```python
from build123d import *

# Parameters (mm, degrees)
SM_BASE_FLANGE_1_DEPTH = 113
EXTRUDE_1_DEPTH        = 4
HOLE_WIZARD_M3_1_D     = 2.5
SKETCH_11_W            = 71.5874944
SKETCH_11_H            = 95.16
CUT_EXTRUDE_1_DEPTH    = 44
HOLE_WIZARD_M3_2_D     = 2.5


# Sheet-metal steps are written as plain solids
with BuildPart() as part:
    # Sketch 2 → 基体-法兰1 (new body)
    with BuildSketch(Plane.XY):
        with BuildLine():
            Line((74, 45.58), (1.5, 45.58))
            ThreePointArc((1.5, 45.58), (0.439339828, 45.140660172), (0, 44.08))
            Line((0, 44.08), (0, -44.08))
            ThreePointArc((0, -44.08), (0.439339828, -45.140660172), (1.5, -45.58))
            Line((1.5, -45.58), (74, -45.58))
            Line((74, -45.58), (74, -47.58))
            Line((74, -47.58), (1.5, -47.58))
            ThreePointArc((1.5, -47.58), (-0.974873734, -46.554873734), (-2, -44.08))
            Line((-2, -44.08), (-2, 44.08))
            ThreePointArc((-2, 44.08), (-0.974873734, 46.554873734), (1.5, 47.58))
            Line((1.5, 47.58), (74, 47.58))
            Line((74, 47.58), (74, 45.58))
        make_face()
    extrude(amount=-SM_BASE_FLANGE_1_DEPTH)

    # 草图7 → 凸台-拉伸1 (add)
    with BuildSketch(Plane.XY):
        with BuildLine():
            Line((74, 45.58), (1.5, 45.58))
            ThreePointArc((1.5, 45.58), (0.439339828, 45.140660172), (0, 44.08))
            Line((0, 44.08), (0, -44.08))
            ThreePointArc((0, -44.08), (0.439339828, -45.140660172), (1.5, -45.58))
            Line((1.5, -45.58), (74, -45.58))
            Line((74, -45.58), (74, 45.58))
        make_face()
    extrude(amount=-EXTRUDE_1_DEPTH)

    # M3 螺纹孔1 (through all)
    with Locations(Plane(origin=(0, 47.58, 0), x_dir=(1, 0, 0), z_dir=(0, 1, 0))):
        with Locations((53.7, 100.6), (66.2, 100.6)):
            Hole(HOLE_WIZARD_M3_1_D / 2)

    # 草图11 → 切除-拉伸1 (cut)
    with BuildSketch(Plane.ZY.offset(2)):
        with Locations((-91.7937472, 0)):
            Rectangle(SKETCH_11_W, SKETCH_11_H)
    extrude(amount=-CUT_EXTRUDE_1_DEPTH, mode=Mode.SUBTRACT)

    # M3 螺纹孔2 (through all)
    with Locations(Plane(origin=(0, 0, -4), x_dir=(-1, 0, 0), z_dir=(0, 0, -1))):
        with Locations((-51.5, 12.5), (-26.5, 12.5), (-26.5, -12.5), (-51.5, -12.5)):
            Hole(HOLE_WIZARD_M3_2_D / 2)


solid = part.part
```
Can you work these out from the model? Positions are in its coordinate system, mm. A direction names the side the tool comes from. Round coordinates to 2 decimals unless told otherwise and drop trailing zeros. Loops run counter-clockwise (first coordinate to the right, second up) from the corner with the lowest first, then second, coordinate; pieces in that order, holes last.
Item 1: If we mould it in two halves opening along X, with no side actions, what happens to faces 4 (the flat face through (74, 0, -2)), 5 (the cylindrical face through (65.623, 46.566, -99.491)), 6 (the cylindrical face through (-1, 46.53, -27.61))? For each: +X half, -X half, draft (parallel to the pull), parting line (faces both ways), or undercut.
Item 2: Suppose I cut it at C-C, the plane y = -39. Write out the boundary of the cut face in (x, z), then the cut area to 3 significant figures.
Item 3: Suppose I cut it at D-D, the plane x = 3. Write out the boundary of the cut face in (y, z).
Item 4: Which directions (+Z, -Z, +X, -X, +Y, -Y) give clear straight access to the entire face, cutting with the end or side of a thin tool? Please do faces 1 (the flat face through (36, 1, -4)), 2 (the flat face through (35, 1, 0)), 3 (the flat face through (-1, 0, -56)).
Item 5: Suppose I cut it at A-A, the plane z = -51. Write out the boundary of the cut face in (x, y), then the cut area to 3 significant figures.
Item 6: Please list where these lines run through material, in increasing order: L1, parallel to Y at x = 51.5, z = -2.7; L2, parallel to Y at x = 28.5, z = -26.5; L3, parallel to X at y = -46.5, z = -100.6.
Item 7: Will these pins go through, and if not, where does the flat tip stop? pin 1 Ø4 at (y, z) = (-15.5, -12) entering from +X; pin 2 Ø1.5 at (x, y) = (66, 14.5) entering from -Z; pin 3 Ø0.6 at (y, z) = (47, -72.5) entering from -X; pin 4 Ø4 at (x, z) = (53.7, -100.6) entering from +Y.
Item 8: Suppose I cut it at B-B, the plane x = 63. Write out the boundary of the cut face in (y, z).
Reported:
1. face 4: +X half
1. face 5: undercut
1. face 6: -X half
2. outline: (-2, -56) - (0, -56) - (0, -4) - (74, -4) - (74, 0) - (-2, 0) - close
2. area: 408 mm2
3. outline: (-47.58, -56) - (-45.58, -56) - (-45.58, -4) - (45.58, -4) - (45.58, -56) - (47.58, -56) - (47.58, 0) - (-47.58, 0) - close
4. face 1: -Z, +X
4. face 2: +Z, +X, -X, +Y, -Y
4. face 3: -Z, -X, +Y, -Y
5. outline: (-2, -44.08) arc R3.5 ccw to (1.5, -47.58) - (74, -47.58) - (74, -45.58) - (1.5, -45.58) arc R1.5 cw to (0, -44.08) - (0, 44.08) arc R1.5 cw to (1.5, 45.58) - (74, 45.58) - (74, 47.58) - (1.5, 47.58) arc R3.5 ccw to (-2, 44.08) - close
5. area: 482 mm2
6. L1: y = -47.58 to -13.75, -11.25 to 11.25, 13.75 to 47.58
6. L2: y = -47.58 to -45.58, 45.58 to 47.58
6. L3: x = 42 to 52.45, 54.95 to 64.95, 67.45 to 74
7. pin 1: stops at x = 0
7. pin 2: stops at z = -4
7. pin 3: stops at x = 42
7. pin 4: stops at y = 47.58
8. outline: (-47.58, -113) - (-45.58, -113) - (-45.58, -4) - (45.58, -4) - (45.58, -113) - (47.58, -113) - (47.58, 0) - (-47.58, 0) - close
